from build123d import *

# Parameters (mm, degrees)
SKETCH_1_R      = 1.5
SKETCH_1_R_2    = 2.1
EXTRUDE_1_DEPTH = 950
FILLET_1_R      = 1


with BuildPart() as part:
    # 草图1 → 凸台-拉伸1 (new body)
    with BuildSketch(Plane.XY):
        Polygon((-10, 10), (-10, 4.8), (-8.34, 3.14), (-8.34, 5.4), (-5.753553391, 5.4), (-3.8, 3.446446609), (-3.8, -3.446446609), (-5.753553391, -5.4), (-8.34, -5.4), (-8.34, -3.14), (-10, -4.8), (-10, -10), (-4.8, -10), (-3.14, -8.34), (-5.4, -8.34), (-5.4, -5.753553391), (-3.446446609, -3.8), (3.446446609, -3.8), (5.4, -5.753553391), (5.4, -8.34), (3.14, -8.34), (4.8, -10), (10, -10), (10, -4.8), (8.34, -3.14), (8.34, -5.4), (5.753553391, -5.4), (3.8, -3.446446609), (3.8, 3.446446609), (5.753553391, 5.4), (8.34, 5.4), (8.34, 3.14), (10, 4.8), (10, 10), (4.8, 10), (3.14, 8.34), (5.4, 8.34), (5.4, 5.753553391), (3.446446609, 3.8), (-3.446446609, 3.8), (-5.4, 5.753553391), (-5.4, 8.34), (-3.14, 8.34), (-4.8, 10), align=None)
        with Locations(Location((-7.5, 7.5, 0), (0, 0, 180))):
            Circle(SKETCH_1_R, mode=Mode.SUBTRACT)
        with Locations(Location((0, 0, 0), (0, 0, 180))):
            Circle(SKETCH_1_R_2, mode=Mode.SUBTRACT)
        with Locations(Location((-7.5, -7.5, 0), (0, 0, 180))):
            Circle(SKETCH_1_R, mode=Mode.SUBTRACT)
        with Locations(Location((7.5, -7.5, 0), (0, 0, 180))):
            Circle(SKETCH_1_R, mode=Mode.SUBTRACT)
        with Locations(Location((7.5, 7.5, 0), (0, 0, 180))):
            Circle(SKETCH_1_R, mode=Mode.SUBTRACT)
    extrude(amount=EXTRUDE_1_DEPTH)

    # 圆角1
    fillet_1_edges = [part.edges().sort_by_distance(p)[0] for p in [
        (10, 10, 475),
        (10, -10, 475),
        (-10, -10, 475),
        (-10, 10, 475),
    ]]
    fillet(fillet_1_edges, radius=FILLET_1_R)


solid = part.part
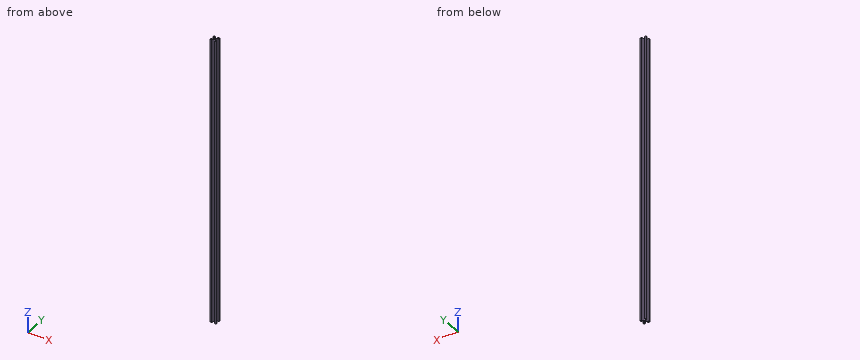
Geometry: final body of the model. Coordinates: model frame, mm. Round coordinates to 2 decimals unless told otherwise and drop trailing zeros. One line per question, with ' | ' between items.
(1) Cut plane A-A on z = 97. Give the number of separate pieces and of enclosed holes in the cut face, plus the area to 3 significant figures.
Check result:
separate pieces: 1 | enclosed holes: 5 | area: 123 mm2
(2) Material intervals for line 1 along Y through (x, z) = (7.5, 739); line 2 along Y through (x, z) = (0, 340.5), sorted ascending. Write a range as from..to.
Check result:
line 1: y = -10..-9, -6..-5.4, 5.4..6, 9..10 | line 2: y = -3.8..-2.1, 2.1..3.8
(3) Contact query for flat-ended pins moving along their axis: P1, Ø2, axis at y = 1, z = 289, coming from the +X side; P2, Ø7.5, axis at x = 0.5, z = 629, coming from the +Y side; P3, Ø2, axis at x = -1.5, z = 775, coming from the -Y side. Output: stop coordinate, or through.
Check result:
P1: stops at x = 3.8 | P2: stops at y = 9.45 | P3: stops at y = -3.8
